Build history of the part. All positions in model axes, mm. Face numbers are marked on the shaded views. A direction names the side the tool comes from. Round coordinates to 2 decimals unless told otherwise and drop trailing zeros. Loops run counter-clockwise (first coordinate to the right, second up) from the corner with the lowest first, then second, coordinate; pieces in that order, holes last. Notation, with made-up numbers: (1.25, 30.25) - (38.25, 30.25) arc R33 ccw to (38.25, 68.25) - close; hole circle Ø11 at (72, 81). An arc over 180 degrees is marked (long way). Use one line per item in the form item = value. Start each with the question number.
Q1. 3-axis set-ups, long thin cutter, end or side, ignore diameter. For the marked faces 1, 2 and 3: which of +Z, -Z, +X, -X, +Y, -Y reach the whole face in a straight line?
Q2. Saw through at D-D (y = 3). Give the cut face in (x, z) (3 decimals).
Q3. Drill centre lines: line 1 (X direction, y = -0.5, z = 42); line 2 (Z direction, x = 12.5, y = -4.25); line 3 (Z direction, x = 4.25, y = -5). Where is each one in solid material? Low to high.
Q4. Saw through at C-C (x = 4). Give the cut face in (y, z).
Q5. Mould opens along Z. For the marked faces 4, 5, 6 and 7 say: released by +Z, released by -Z, zero draft, split by the parting line, or undercut.
Q6. Saw through at A-A (z = 0). Give the cut face in (x, y) (3 decimals), then the cut area to 3 significant figures.
Q7. Saw through at B-B (y = -5.5). Give the cut face in (x, z).
Q8. Pin check, flat tips, straight feed: pin 1 (2.5 mm diameter, centred on x = -2.5, z = 9, fed in from -Y); pin 2 (1 mm diameter, centred on x = -13.5, z = 42.5, fed in from -Y); pin 3 (1.8 mm diameter, centred on x = 10, z = -1.5, fed in from -Y). Stop position of each tip, or through.
```python
from build123d import *

# Parameters (mm, degrees)
BOSS_EXTRU_1_DEPTH                                = 4
ESQUISSE2_R                                       = 1.15
ENL_V_MAT_EXTRU_1_DEPTH                           = 18.663521733
CHAMBRAGE_POUR_VIS_SIX_PANS_CREUX_M21_D           = 2.2
CHAMBRAGE_POUR_VIS_SIX_PANS_CREUX_M21_CBORE_D     = 4.4
CHAMBRAGE_POUR_VIS_SIX_PANS_CREUX_M21_CBORE_DEPTH = 4
BOSS_EXTRU_2_DEPTH                                = 28
COQUE1_START                                      = -12
COQUE1_DEPTH                                      = 24
COQUE1_START_2                                    = -51.994775807
COQUE1_2_DEPTH                                    = 48.056615462
ENL_V_MAT_EXTRU_2_DEPTH                           = 11
ESQUISSE8_W                                       = 15
ESQUISSE8_H                                       = 5
ENL_V_MAT_EXTRU_3_DEPTH                           = 63


with BuildPart() as part:
    # Esquisse1 → Boss.-Extru.1 (new, symmetric)
    with BuildSketch(Plane.XY):
        Polygon((-14, 2), (-7.85, 2), (-7.85, 8.2), (4.95, 8.2), (7.85, 5.6), (7.85, 2), (14, 2), (14, 12), (-14, 12), align=None)
    extrude(amount=BOSS_EXTRU_1_DEPTH, both=True)

    # Esquisse2 → Enlèv. mat.-Extru.1 (cut, through all)
    with BuildSketch(Plane.XZ.offset(-2)):
        with Locations((10.925, 0)):
            Circle(ESQUISSE2_R)
        with Locations(Location((-10.925, 0, 0), (0, 0, 180))):
            Circle(ESQUISSE2_R)
    extrude(amount=-ENL_V_MAT_EXTRU_1_DEPTH, mode=Mode.SUBTRACT)

    # Chambrage pour vis à six pans creux M21 (through all)
    with Locations(Plane(origin=(0, 12, 0), x_dir=(1, 0, 0), z_dir=(0, 1, 0))):
        with Locations((-10.925, 0), (10.925, 0)):
            CounterBoreHole(CHAMBRAGE_POUR_VIS_SIX_PANS_CREUX_M21_D / 2, CHAMBRAGE_POUR_VIS_SIX_PANS_CREUX_M21_CBORE_D / 2, CHAMBRAGE_POUR_VIS_SIX_PANS_CREUX_M21_CBORE_DEPTH)

    # Esquisse6 → Boss.-Extru.2 (add)
    with BuildSketch(Plane.ZY.offset(14)):
        Polygon((4.5, 2), (4, 2), (4, 12), (14, 12), (54, 1), (54, -7), (4.5, -7), align=None)
    extrude(amount=-BOSS_EXTRU_2_DEPTH)

    # Chanfrein1
    # the kernel refuses this chamfer: 3 mm, written as the material it takes off along each edge
    with BuildSketch(Plane(origin=(-19.957306113, 1, 54), x_dir=(0, 0.2651564830210424, -0.9642053928037904), z_dir=(1, 0, 0))) as chanfrein1_piece_1:
        with BuildLine():
            Line((2.381812022, 0.07273839), (-0.701687646, -2.277268941))
            Line((-0.701687646, -2.277268941), (-0.75953997, -2.261359552))
            ThreePointArc((-0.75953997, -2.261359552), (-0.373628773, -1.132368609), (-0.057852324, 0.015909389))
            Line((-0.057852324, 0.015909389), (0, 0.06))
            ThreePointArc((0, 0.06), (1.190906011, 0.06), (2.381812022, 0.13273839))
            Line((2.381812022, 0.13273839), (2.381812022, 0.07273839))
        make_face()
    extrude(amount=39.914612227, mode=Mode.SUBTRACT)
    with BuildSketch(Plane(origin=(14, 15.477681924, 1.353883912), x_dir=(-1, 0, 0), z_dir=(0, -0.26515648302104217, 0.9642053928037905))) as chanfrein1_piece_2:
        with BuildLine():
            Line((3.084852814, -0.084852814), (-0.084852814, 3.084852814))
            Line((-0.084852814, 3.084852814), (-0.144852814, 3.084852814))
            ThreePointArc((-0.144852814, 3.084852814), (-0.06, 1.542426407), (-0.06, 0))
            Line((-0.06, 0), (0, -0.06))
            ThreePointArc((0, -0.06), (1.542426407, -0.06), (3.084852814, -0.144852814))
            Line((3.084852814, -0.144852814), (3.084852814, -0.084852814))
        make_face()
    extrude(amount=62.315569228, mode=Mode.SUBTRACT)
    with BuildSketch(Plane(origin=(-15.310375108, 12, 14), x_dir=(0, 0, -1), z_dir=(1, 0, 0))) as chanfrein1_piece_3:
        with BuildLine():
            Line((0.523904139, 0.016053697), (-0.509407938, -0.123437518))
            Line((-0.509407938, -0.123437518), (-0.525317327, -0.065585195))
            ThreePointArc((-0.525317327, -0.065585195), (-0.268484987, -0.011605966), (-0.015909389, 0.057852324))
            Line((-0.015909389, 0.057852324), (0, 0.06))
            ThreePointArc((0, 0.06), (0.261952069, 0.06), (0.523904139, 0.076053697))
            Line((0.523904139, 0.076053697), (0.523904139, 0.016053697))
        make_face()
    extrude(amount=30.620750216, mode=Mode.SUBTRACT)
    with BuildSketch(Plane(origin=(-14, 15.477681924, 1.353883912), x_dir=(1, 0, 0), z_dir=(0, -0.26515648302104217, 0.9642053928037905))) as chanfrein1_piece_4:
        with BuildLine():
            Line((3.084852814, 0.084852814), (-0.084852814, -3.084852814))
            Line((-0.084852814, -3.084852814), (-0.144852814, -3.084852814))
            ThreePointArc((-0.144852814, -3.084852814), (-0.06, -1.542426407), (-0.06, 0))
            Line((-0.06, 0), (0, 0.06))
            ThreePointArc((0, 0.06), (1.542426407, 0.06), (3.084852814, 0.144852814))
            Line((3.084852814, 0.144852814), (3.084852814, 0.084852814))
        make_face()
    extrude(amount=62.315569228, mode=Mode.SUBTRACT)

    # Coque1: read off the stored shape, not the designer's step
    # Coque1 outline → Coque1 (cut)
    with BuildSketch(Plane.YZ.offset(COQUE1_START)):
        Polygon((-7, 5.5), (10, 5.5), (10, 13.460632375), (9.928572392, 13.989748207), (-0.143118288, 50.614077951), (-1.961619074, 52), (-7, 52), align=None)
    extrude(amount=COQUE1_DEPTH, mode=Mode.SUBTRACT)

    # Coque1 2 outline → Coque1 2 (add)
    with BuildSketch(Plane(origin=(0, 0, 0), x_dir=(1, 0, 0), z_dir=(0, 0.26515648302104255, -0.9642053928037904)).offset(COQUE1_START_2)):
        Polygon((12, -11.454228351), (10.171572875, -13.282655476), (12, -13.282655476), align=None)
        Polygon((-10.171572875, -13.282655476), (-12, -11.454228351), (-12, -13.282655476), align=None)
    extrude(amount=COQUE1_2_DEPTH)

    # Esquisse7 → Enlèv. mat.-Extru.2 (cut)
    with BuildSketch(Plane(origin=(0, 0, -4), x_dir=(-1, 0, 0), z_dir=(0, 0, -1))):
        Polygon((-12, 2), (-12, -7), (12, -7), (12, 2), (7.85, 2), (-7.85, 2), align=None)
        Polygon((-7.85, 2), (7.85, 2), (7.85, 8.2), (-4.95, 8.2), (-7.85, 5.6), align=None)
    extrude(amount=-ENL_V_MAT_EXTRU_2_DEPTH, mode=Mode.SUBTRACT)

    # Esquisse8 → Enlèv. mat.-Extru.3 (cut, through all)
    with BuildSketch(Plane(origin=(14, 0, 0), x_dir=(0, 0, -1), z_dir=(1, 0, 0))):
        with Locations((-41.5, -4.5)):
            Rectangle(ESQUISSE8_W, ESQUISSE8_H)
    extrude(amount=-ENL_V_MAT_EXTRU_3_DEPTH, mode=Mode.SUBTRACT)


solid = part.part
```
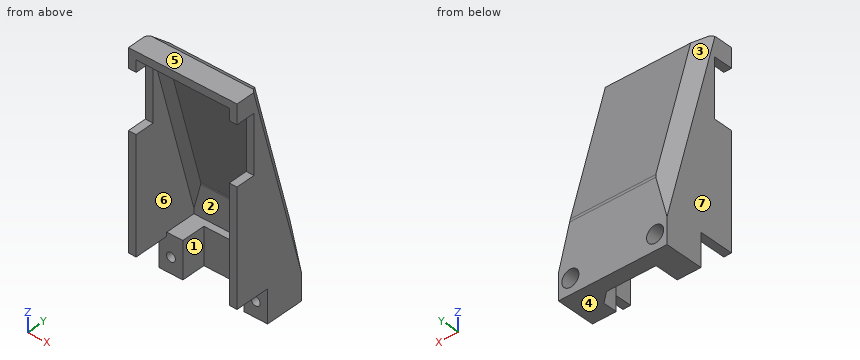
Report:
q1.face_1 = -Z, -Y
q1.face_2 = -Y
q1.face_3 = +Z, -X, +Y
q2.outline = (-14, -4) - (-7.85, -4) - (-7.85, 5.5) - (-12, 5.5) - (-12, 32.289) - (-10.172, 39.185) - (10.172, 39.185) - (12, 32.289) - (12, 5.5) - (7.85, 5.5) - (7.85, -4) - (14, -4) - (14, 35.413) - (11, 46.727) - (-11, 46.727) - (-14, 35.413) - close; hole circle Ø2.3 at (-10.925, 0); hole circle Ø2.3 at (10.925, 0)
q3.line_1 = -14 to -12, 12 to 14
q3.line_2 = 4.5 to 34, 49 to 54
q3.line_3 = 52 to 54
q4.outline = (-7, 52) - (-1.96, 52) - (-0.14, 50.61) - (9.93, 13.99) - (10, 13.46) - (10, 5.5) - (8.2, 5.5) - (8.2, -4) - (12, -4) - (12, 13.6) - (11.89, 14.39) - (1.61, 51.8) - (-1.29, 54) - (-7, 54) - close
q5.face_4 = released by -Z
q5.face_5 = released by +Z
q5.face_6 = undercut
q5.face_7 = zero draft
q6.outline = (-14, 2) - (-12.075, 2) - (-12.075, 8) - (-13.125, 8) - (-13.125, 12) - (-14, 12) - close; (-9.775, 2) - (-7.85, 2) - (-7.85, 8.2) - (4.95, 8.2) - (7.85, 5.6) - (7.85, 2) - (9.775, 2) - (9.775, 8) - (8.725, 8) - (8.725, 12) - (-8.725, 12) - (-8.725, 8) - (-9.775, 8) - close; (12.075, 2) - (14, 2) - (14, 12) - (13.125, 12) - (13.125, 8) - (12.075, 8) - close
q6.area = 124 mm²
q7.outline = (-14, 4.5) - (-12, 4.5) - (-12, 34) - (-14, 34) - close; (-14, 49) - (-12, 49) - (-12, 52) - (12, 52) - (12, 49) - (14, 49) - (14, 54) - (-14, 54) - close; (12, 4.5) - (14, 4.5) - (14, 34) - (12, 34) - close
q8.pin_1 = 10
q8.pin_2 = -2
q8.pin_3 = 2
